Geometry check sheet. Reference: the model listing, model coordinates, mm. A direction names the side the tool comes from. Coordinates: 2 decimals unless noted, no trailing zeros. One line per item, written item: value.
from build123d import *

# Parameters (mm, degrees)
SKETCH1_R               = 34.1
BOSS_EXTRUDE1_DEPTH     = 1.75
SKETCH4_R               = 28.5
BOSS_EXTRUDE2_DEPTH     = 2
CUT_EXTRUDE2_DEPTH      = 49.351525312
CUT_EXTRUDE2_DEPTH_BACK = 49.351525312
SKETCH3_R               = 2.25
CUT_EXTRUDE1_DEPTH      = 49.351525312
CUT_EXTRUDE1_DEPTH_BACK = 49.351525312
SKETCH2_R               = 7.25
FILLET1_R               = 0.5


with BuildPart() as part:
    # Sketch1 → Boss-Extrude1 (new, symmetric)
    with BuildSketch(Plane.XY):
        Circle(SKETCH1_R)
    extrude(amount=BOSS_EXTRUDE1_DEPTH, both=True)

    # Sketch4 → Boss-Extrude2 (add)
    with BuildSketch(Plane.XY.offset(1.75)):
        Circle(SKETCH4_R)
    extrude(amount=BOSS_EXTRUDE2_DEPTH)

    # Sketch3 → Cut-Extrude2 (cut, two sides: drawn at the far end of the back side and taken through both)
    with BuildSketch(Plane.XY.offset(1.75).offset(-CUT_EXTRUDE2_DEPTH_BACK)):
        with Locations((0, 24.75)):
            Circle(SKETCH3_R)
        with Locations((0, 11.3137085)):
            Circle(SKETCH3_R)
        with Locations((24.75, 0)):
            Circle(SKETCH3_R)
        with Locations((11.3137085, 0)):
            Circle(SKETCH3_R)
        with Locations((0, -24.75)):
            Circle(SKETCH3_R)
        with Locations((0, -11.3137085)):
            Circle(SKETCH3_R)
        with Locations((-24.75, 0)):
            Circle(SKETCH3_R)
        with Locations((-11.3137085, 0)):
            Circle(SKETCH3_R)
    extrude(amount=CUT_EXTRUDE2_DEPTH + CUT_EXTRUDE2_DEPTH_BACK, mode=Mode.SUBTRACT)

    # Sketch2 → Cut-Extrude1 (cut, two sides: drawn at the far end of the back side and taken through both)
    with BuildSketch(Plane.XY.offset(1.75).offset(-CUT_EXTRUDE1_DEPTH_BACK)):
        Circle(SKETCH2_R)
    extrude(amount=CUT_EXTRUDE1_DEPTH + CUT_EXTRUDE1_DEPTH_BACK, mode=Mode.SUBTRACT)

    # Fillet1
    fillet1_edges = [part.edges().sort_by_distance(p)[0] for p in [
        (-28.5, 0, 3.75),
    ]]
    fillet(fillet1_edges, radius=FILLET1_R)


solid = part.part
(1) Material ranges on probe 1 along Y at (x, z) = (0, -0.1); probe 2 along Z at (x, y) = (17, 28); probe 3 along Y at (x, z) = (-1, -0.3), recorded low to high. Write a range as from..to.
Reply:
probe 1: -34.1..-27, -22.5..-13.56, -9.06..-7.25, 7.25..9.06, 13.56..22.5, 27..34.1
probe 2: -1.75..1.75
probe 3: -34.09..-26.77, -22.73..-13.33, -9.3..-7.18, 7.18..9.3, 13.33..22.73, 26.77..34.09
(2) Go/stop test with a flat-tipped pin: pin 1 Ø23 at (x, y) = (0, 0) entering from -Z. Record where the tip stops, or that it passes through.
Reply:
pin 1: z = -1.75
(3) Release check for a two-part mould opening along X. For faces 3 (the face through (3.35, -6.43, 0.96)), 4 (the face through (-4.44, 33.81, 0.02)), 5 (the face through (0, 8, -1.75)) record: pulls with the +X half, pulls with the -X half, needs draft (parallel to the pull), parting line crosses it, or undercut.
Reply:
face 3: undercut
face 4: parting line crosses it
face 5: needs draft
(4) Cross-section at A-A on x = 0. State how many separate pieces and enclosed holes the cut face has, and give its area (3 significant figures).
Reply:
separate pieces: 6
enclosed holes: 0
area: 174 mm2
(5) Access from +Z, -Z, +X, -X, +Y, -Y to the whole of each face (thin tool, end or side, straight path). Record for faces 1 (the face through (26.327, -10.916, 2.49)), 2 (the face through (0, -27, 1)).
Reply:
face 1: +Z
face 2: +Z, -Z
